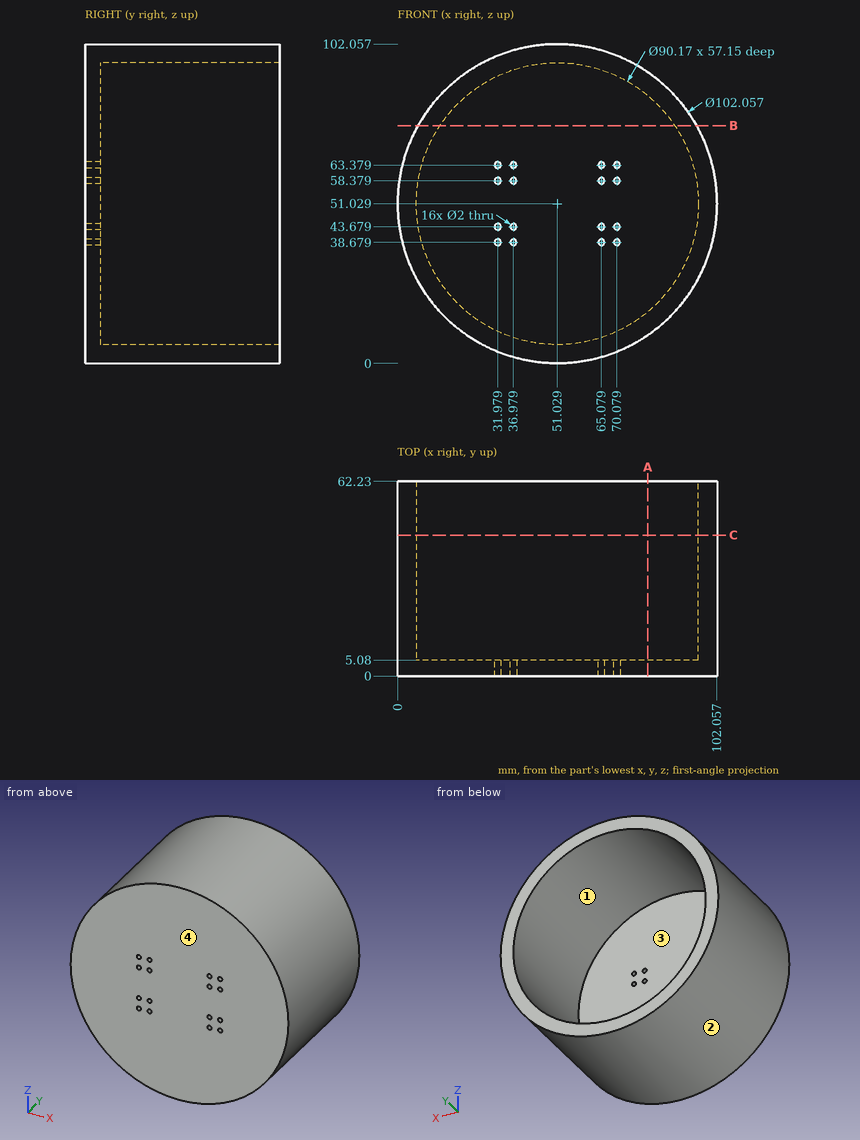
Can you work these out from the drawing? Everything is in mm from the part's minimum corner. Round coordinates to 2 decimals unless told otherwise and drop trailing zeros. Loops run counter-clockwise (first coordinate to the right, second up) from the corner with the lowest first, then second, coordinate; pieces in that order, holes last. Notation, with made-up numbers: (84, 66.5) -> (138, 66.5) arc R14 cw to (138, 77.5) -> close; hole circle Ø5 at (-25, 68). An arc over 180 degrees is marked (long way). Put each result on its own line as item: value.
Q1. I want a section at A-A on x = 80. Write out the boundary of the cut face in (y, z) (1 decimal), and give its area (3 significant figures).
Checks:
outline: (0, 9) -> (62.2, 9) -> (62.2, 16.5) -> (5.1, 16.5) -> (5.1, 85.6) -> (62.2, 85.6) -> (62.2, 93) -> (0, 93) -> close
area: 1,280 mm2
Q2. For pin 1 Ø3 at (y, z) = (55, 77.5) entering from -X; pin 2 Ø3 at (x, z) = (76.5, 53.5) entering from +Y; pin 3 Ø1.8 at (x, z) = (36.98, 43.68) entering from -Y; pin 4 Ø2 at (x, y) = (38.5, 50) entering from +Z, each with a flat end and sliding along its axis, tell me the tip position at first contact or that it passes through.
Checks:
pin 1: x = 6.53
pin 2: y = 5.08
pin 3: through
pin 4: z = 100.74
Q3. Thinking about a two-plate mould opening in Z: for the marked faces 1, 2, 3 and 4, which applies, pulls with the +Z half, pulls with the -Z half, needs draft (parallel to the pull), parting line crosses it, or undercut?
Checks:
face 1: undercut
face 2: parting line crosses it
face 3: undercut
face 4: needs draft
Q4. Please list where these lines run through material, in increasing order: line 1 (Y direction, x = 69, z = 50); line 2 (X direction, y = 56, z = 21) (1 decimal); line 3 (Z direction, x = 19, y = 6.5) (1 decimal). Write a range as from..to.
Checks:
line 1: 0..5.08
line 2: 9.8..17.4, 84.7..92.3
line 3: 11.3..19.3, 82.8..90.8
Q5. I want a section at B-B on z = 76. Write out the boundary of the cut face in (x, y), and give its area (3 significant figures).
Checks:
outline: (6.53, 0) -> (95.53, 0) -> (95.53, 62.23) -> (88.57, 62.23) -> (88.57, 5.08) -> (13.49, 5.08) -> (13.49, 62.23) -> (6.53, 62.23) -> close
area: 1,250 mm2
Q6. I want a section at C-C on y = 45. Write out the boundary of the cut face in (x, z) (1 decimal).
Checks:
outline: circle Ø102.1 at (51, 51); hole circle Ø90.2 at (51, 51)
